Here's the drawing with two shaded views (mm, measured from the low corner). I have some questions. A direction names the side the tool comes from. Give positions to 0.01 mm unless a question says otherwise; leave off trailing zeros. Write each loop counter-clockwise with the first axis right and the second up, starting at its lowest first coordinate (ties: lowest second). Pieces come first, ordered by that corner, then holes. Notation, with made-up numbers: M 46.5,-34 L 83.5,-34 A31 ccw 83.5,-2 Z; hole C 10,6.5 d1. An arc over 180 degrees is marked long. Answer as a JSON object with one key per item and string values. Group by question number.
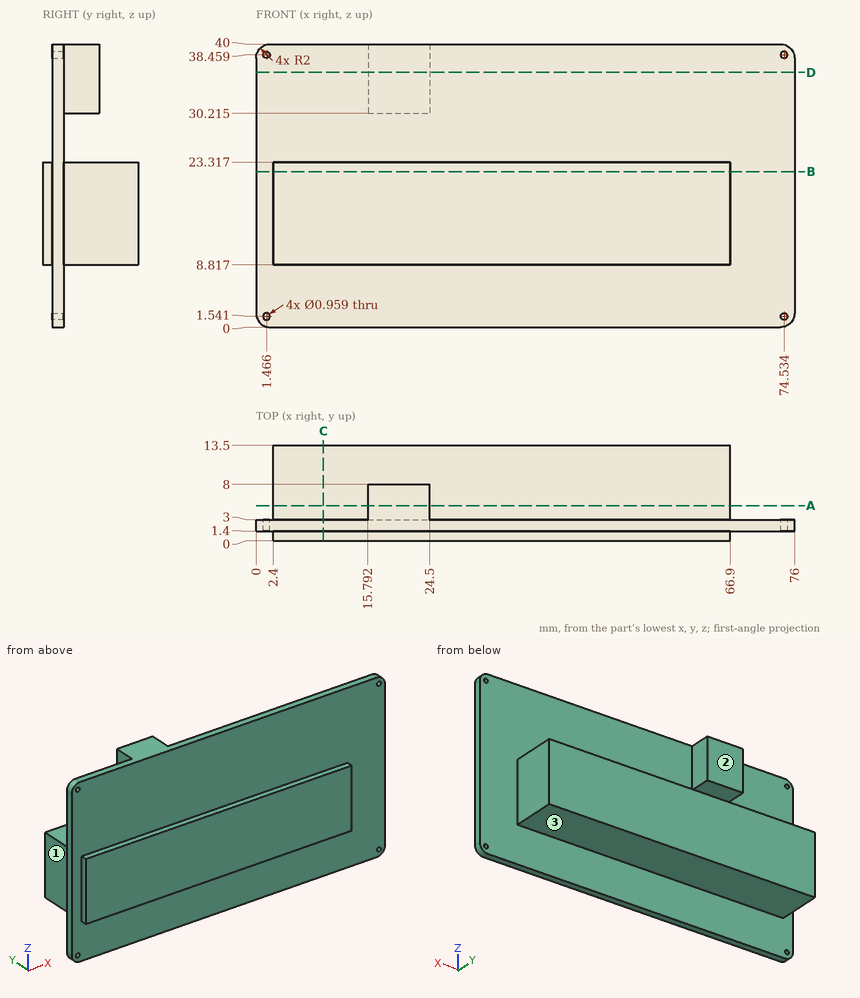
1) If we section it at C-C, the plane x = 9.5: List the corners of the cut face in (y, z) for me.
2) For the marked faces 1, 2 and 3, which set-ups out of +Z, -Z, +X, -X, +Y, -Y let a thin tool reach every point of the face, with its end or its side?
3) If we section it at B-B, the plane z = 22: List the corners of the cut face in (x, y) for me.
4) Please list where these lines run through material, in increasing order: line 1 along Y through (x, z) = (32, 27); line 2 along Z through (x, y) = (25, 11.5); line 3 along X through (y, z) = (13.25, 13). Write a range as from..to.
5) If we section it at D-D, the plane z = 36: List the corners of the cut face in (x, y) for me.
6) I'm going to push flat-ended pins straight in: pin 1 (2.5 mm diameter, centred on y = 5, z = 34, fed in from +X); pin 2 (4 mm diameter, centred on y = 6.5, z = 35.5, fed in from -X); pin 3 (1.5 mm diameter, centred on x = 43.5, y = 9, fed in from +Z). Where does each tip first touch, or does it pass through?
7) If we section it at A-A, the plane y = 5: List the corners of the cut face in (x, z) for me (1 decimal), plus the area to 3 significant figures.
Taken from the geometry:
{
 "1": {"outline": "M 0,8.82 L 1.4,8.82 L 1.4,0 L 3,0 L 3,8.82 L 13.5,8.82 L 13.5,23.32 L 3,23.32 L 3,40 L 1.4,40 L 1.4,23.32 L 0,23.32 Z"},
 "2": {"face 1": "+Z, -Z, -X, +Y", "face 2": "+Z, +X, -X, +Y", "face 3": "-Z, +X, -X, +Y"},
 "3": {"outline": "M 0,1.4 L 2.4,1.4 L 2.4,0 L 66.9,0 L 66.9,1.4 L 76,1.4 L 76,3 L 66.9,3 L 66.9,13.5 L 2.4,13.5 L 2.4,3 L 0,3 Z"},
 "4": {"line 1": "1.4..3", "line 2": "8.82..23.32", "line 3": "2.4..66.9"},
 "5": {"outline": "M 0,1.4 L 76,1.4 L 76,3 L 24.5,3 L 24.5,8 L 15.79,8 L 15.79,3 L 0,3 Z"},
 "6": {"pin 1": "x = 24.5", "pin 2": "x = 15.79", "pin 3": "z = 23.32"},
 "7": {"outline": "M 2.4,8.8 L 66.9,8.8 L 66.9,23.3 L 2.4,23.3 Z; M 15.8,30.2 L 24.5,30.2 L 24.5,40 L 15.8,40 Z", "area": "1,020 mm²"}
}
